Here's how the part is built. I have some questions about the finished solid (model axes, mm). Coordinates: 2 decimals unless noted, no trailing zeros. Write each loop counter-clockwise with the first axis right and the second up, starting at its lowest first coordinate (ties: lowest second). Pieces come first, ordered by that corner, then holes.
from build123d import *

# Parameters (mm, degrees)
ESBO_O1_R                = 2.79
RESSALTO_EXTRUS_O1_DEPTH = 120


with BuildPart() as part:
    # Esboço1 → Ressalto-extrusão1 (new body)
    with BuildSketch(Plane(origin=(0, 85, 0), x_dir=(1, 0, 0), z_dir=(0, 1, 0))):
        with BuildLine():
            Line((6.162658774, -1.825961894), (7.216878365, 0))
            Line((7.216878365, 0), (6.162658774, 1.825961894))
            ThreePointArc((6.162658774, 1.825961894), (4.113620668, 2.375), (4.662658774, 4.424038106))
            Line((4.662658774, 4.424038106), (3.608439182, 6.25))
            Line((3.608439182, 6.25), (1.5, 6.25))
            ThreePointArc((1.5, 6.25), (0, 4.75), (-1.5, 6.25))
            Line((-1.5, 6.25), (-3.608439182, 6.25))
            Line((-3.608439182, 6.25), (-4.662658774, 4.424038106))
            ThreePointArc((-4.662658774, 4.424038106), (-4.113620668, 2.375), (-6.162658774, 1.825961894))
            Line((-6.162658774, 1.825961894), (-7.216878365, 0))
            Line((-7.216878365, 0), (-6.162658774, -1.825961894))
            ThreePointArc((-6.162658774, -1.825961894), (-4.113620668, -2.375), (-4.662658774, -4.424038106))
            Line((-4.662658774, -4.424038106), (-3.608439182, -6.25))
            Line((-3.608439182, -6.25), (-1.5, -6.25))
            ThreePointArc((-1.5, -6.25), (0, -4.75), (1.5, -6.25))
            Line((1.5, -6.25), (3.608439182, -6.25))
            Line((3.608439182, -6.25), (4.662658774, -4.424038106))
            ThreePointArc((4.662658774, -4.424038106), (4.113620668, -2.375), (6.162658774, -1.825961894))
        make_face()
        with Locations(Location((0, 0, 0), (0, 0, 90))):
            Circle(ESBO_O1_R, mode=Mode.SUBTRACT)
    extrude(amount=-RESSALTO_EXTRUS_O1_DEPTH)


solid = part.part
1. If I drill on line 1 (X direction, y = 51, z = 0); line 2 (X direction, y = 75.5, z = -1.5); line 3 (X direction, y = 33.5, z = -4.25), over which ranges is the centre line in solid material (lowest first)?
2. I want a section at A-A (x = 0). List the corners of the cut face in (y, z) for me, then the cut area to 3 significant figures.
3. For pin 1 Ø1.5 at (x, y) = (-5, -11) entering from -Z; pin 2 Ø3 at (y, z) = (4.5, -3.5) entering from -X, each with a flat end and sliding along its axis, tell me the tip position at first contact or that it passes through.
4. I want a section at B-B (y = -11). List the corners of the cut face in (x, z) for me (3 decimals), then the cut area to 3 significant figures.
5. Thinking about a two-plate mould opening in Z: for faces 1 (the face through (4.143, 25.84, -5.324)), 2 (the face through (-4.1, 25.8, -2.4)), 3 (the face through (4.13, 25.84, 5.35)), which applies, pulls with the +Z half, pulls with the -Z half, needs draft (parallel to the pull), parting line crosses it, or undercut?
Response values:
1. line 1: x = -7.22 to -2.79, 2.79 to 7.22
1. line 2: x = -6.35 to -2.35, 2.35 to 6.35
1. line 3: x = -4.42 to 4.42
2. outline: (-35, -4.75) - (85, -4.75) - (85, -2.79) - (-35, -2.79) - close; (-35, 2.79) - (85, 2.79) - (85, 4.75) - (-35, 4.75) - close
2. area: 470 mm2
3. pin 1: stops at z = -5.14
3. pin 2: stops at x = -4.66
4. outline: (-7.217, 0) - (-6.163, -1.826) arc R1.5 cw to (-4.663, -4.424) - (-3.608, -6.25) - (-1.5, -6.25) arc R1.5 cw to (1.5, -6.25) - (3.608, -6.25) - (4.663, -4.424) arc R1.5 cw to (6.163, -1.826) - (7.217, 0) - (6.163, 1.826) arc R1.5 cw to (4.663, 4.424) - (3.608, 6.25) - (1.5, 6.25) arc R1.5 cw to (-1.5, 6.25) - (-3.608, 6.25) - (-4.663, 4.424) arc R1.5 cw to (-6.163, 1.826) - close; hole circle Ø5.58 at (0, 0)
4. area: 89.7 mm2
5. face 1: pulls with the -Z half
5. face 2: undercut
5. face 3: pulls with the +Z half
